Read the model definition and answer for the solid it produces. Units are mm, in the model's axes. A direction names the side the tool comes from. Give positions to 0.01 mm unless a question says otherwise; leave off trailing zeros. Write each loop counter-clockwise with the first axis right and the second up, starting at its lowest first coordinate (ties: lowest second). Pieces come first, ordered by that corner, then holes.
```python
from build123d import *

# Parameters (mm, degrees)
SKETCH1_R           = 2.25
SKETCH1_R_2         = 1
BOSS_EXTRUDE1_DEPTH = 2
SKETCH4_R           = 7
SKETCH4_R_2         = 1
BOSS_EXTRUDE2_DEPTH = 1
SKETCH5_R           = 7
SKETCH5_R_2         = 3.05
BOSS_EXTRUDE3_DEPTH = 4
CUT_EXTRUDE1_DEPTH  = 3


with BuildPart() as part:
    # Sketch1 → Boss-Extrude1 (new, symmetric)
    with BuildSketch(Plane.XY):
        with BuildLine():
            Line((0, 10), (175, 10))
            ThreePointArc((175, 10), (185, 0), (175, -10))
            Line((175, -10), (0, -10))
            ThreePointArc((0, -10), (-10, 0), (0, 10))
        make_face()
        with Locations((175, 0)):
            Circle(SKETCH1_R, mode=Mode.SUBTRACT)
        with Locations((8.098e-06, -5.598e-06)):
            Circle(SKETCH1_R_2, mode=Mode.SUBTRACT)
    extrude(amount=BOSS_EXTRUDE1_DEPTH, both=True)

    # Sketch4 → Boss-Extrude2 (add)
    with BuildSketch(Plane.XY.offset(2)):
        with Locations((8.098e-06, -5.598e-06)):
            Circle(SKETCH4_R)
        with Locations((8.098e-06, -5.598e-06)):
            Circle(SKETCH4_R_2, mode=Mode.SUBTRACT)
    extrude(amount=BOSS_EXTRUDE2_DEPTH)

    # Sketch5 → Boss-Extrude3 (add)
    with BuildSketch(Plane.XY.offset(3)):
        with Locations((8.098e-06, -5.598e-06)):
            Circle(SKETCH5_R)
        with Locations((8.098e-06, -5.598e-06)):
            Circle(SKETCH5_R_2, mode=Mode.SUBTRACT)
    extrude(amount=BOSS_EXTRUDE3_DEPTH)

    # Sketch6 → Cut-Extrude1 (cut)
    with BuildSketch(Plane(origin=(0, 0, -2), x_dir=(-1, 0, 0), z_dir=(0, 0, -1))):
        Polygon((-0.324730573, 2.050263829), (0, 2.374994402), (0.324730573, 2.050261264), (0.733914965, 2.258751125), (0.942404034, 1.849564293), (1.395988428, 1.921405003), (1.46782763, 1.467818534), (1.921412023, 1.395977824), (1.849569238, 0.942391923), (2.25875363, 0.733902061), (2.050261329, 0.324716876), (2.374991902, -1.3697e-05), (2.050258764, -0.324744269), (2.258748625, -0.733928662), (1.849561793, -0.942417731), (1.921402503, -1.396002124), (1.467816034, -1.467841327), (1.395975324, -1.92142572), (0.942389423, -1.849582934), (0.733899561, -2.258767327), (0.324714376, -2.050275026), (-1.6197e-05, -2.375005598), (-0.324746769, -2.05027246), (-0.733931162, -2.258762322), (-0.942420231, -1.84957549), (-1.396004624, -1.9214162), (-1.467843827, -1.467829731), (-1.92142822, -1.395989021), (-1.849585434, -0.94240312), (-2.258769827, -0.733913258), (-2.050277526, -0.324728073), (-2.375008098, 2.5e-06), (-2.05027496, 0.324733073), (-2.258764822, 0.733917465), (-1.84957799, 0.942406534), (-1.9214187, 1.395990928), (-1.467832231, 1.46783013), (-1.395991521, 1.921414523), (-0.94240562, 1.849571738), (-0.733915758, 2.25875613), align=None)
    extrude(amount=-CUT_EXTRUDE1_DEPTH, mode=Mode.SUBTRACT)


solid = part.part
```
Item 1: Find the intervals of material crossed by line 1 along Y through (x, z) = (175, 0.2); line 2 along Z through (x, y) = (85.5, 2.75); line 3 along X through (y, z) = (0.5, 3.75), in increasing order.
Result set:
line 1: y = -10 to -2.25, 2.25 to 10
line 2: z = -2 to 2
line 3: x = -6.98 to -3.01, 3.01 to 6.98
Item 2: Which of the six approach directions +Z, -Z, +X, -X, +Y, -Y give full straight-line access (tool end or side, diameter ignored) to faces 5 (the flat face through (89, -10, 0)), 6 (the flat face through (-1, 1, 3))?
Result set:
face 5: +Z, -Z, +X, -X, -Y
face 6: +Z
Item 3: Section A-A (z = 4.75) is taken. Write down the section's boundary in (x, y), and give its area (3 significant figures).
Result set:
outline: circle Ø14 at (0, 0); hole circle Ø6.1 at (0, 0)
area: 125 mm2
Item 4: Determine the mould class of faces 1 (the cylindrical face through (185, 0, 0)), 2 (the flat face through (1.5, -3, 7)), 3 (the cylindrical face through (-10, 0, 0)), 4 (the cylindrical face through (-2.42, -1.856, 4.972)) for opening direction X: pulls with the +X half, pulls with the -X half, needs draft (parallel to the pull), parting line crosses it, or undercut.
Result set:
face 1: pulls with the +X half
face 2: needs draft
face 3: pulls with the -X half
face 4: undercut
Item 5: Each of these flat-tipped pins is pushed along its axis until it touches: pin 1 Ø2.5 at (x, y) = (0.5, -0.5) entering from -Z; pin 2 Ø10 at (x, y) = (37, -5.5) entering from +Z; pin 3 Ø3 at (x, y) = (0, 0) entering from +Z. Where does it stop, or does it pass through?
Result set:
pin 1: stops at z = 1
pin 2: stops at z = 2
pin 3: stops at z = 3
Item 6: Section C-C (x = 160) is taken. Write down the section's boundary in (y, z).
Result set:
outline: (-10, -2) - (10, -2) - (10, 2) - (-10, 2) - close
Item 7: Section B-B (y = -4.75) is taken. Write down the section's boundary in (x, z).
Result set:
outline: (-8.8, -2) - (183.8, -2) - (183.8, 2) - (5.14, 2) - (5.14, 7) - (-5.14, 7) - (-5.14, 2) - (-8.8, 2) - close
